```python
from build123d import *

# Parameters (mm, degrees)
F0_W     = 69.7
F0_H     = 17.7
F1_DEPTH = 1
F3_W     = 75.7
F3_H     = 23.7
F3_W_2   = 69.7
F3_H_2   = 17.7
F4_DEPTH = 1


with BuildPart() as f1:
    # F0 (on Top) → F1 (new body)
    with BuildSketch(Plane.XY):
        Rectangle(F0_W, F0_H)
    extrude(amount=F1_DEPTH)

    # F3 (on face) → F4 (join)
    with BuildSketch(Plane(origin=(0, 0, 0), x_dir=(1, 0, 0), z_dir=(0, 0, -1))):
        Rectangle(F3_W, F3_H)
        Rectangle(F3_W_2, F3_H_2, mode=Mode.SUBTRACT)
        Rectangle(F3_W_2, F3_H_2)
    extrude(amount=F4_DEPTH)


solid = f1.part
```
Verification items for the finished model (mm, model axes). Round coordinates to 2 decimals unless told otherwise and drop trailing zeros. Order: outer loops, then holes, each group sorted by start corner. A loop starts at its lowest first (then second) coordinate and runs counter-clockwise, first axis right, second up.
1) Cross-section at A-A, the plane x = 4.5. Record the cut outline in (y, z).
Geometry says:
outline: (-11.85, -1) - (11.85, -1) - (11.85, 0) - (8.85, 0) - (8.85, 1) - (-8.85, 1) - (-8.85, 0) - (-11.85, 0) - close
2) Cross-section at B-B, the plane y = 0.25. Record the cut outline in (x, z).
Geometry says:
outline: (-37.85, -1) - (37.85, -1) - (37.85, 0) - (34.85, 0) - (34.85, 1) - (-34.85, 1) - (-34.85, 0) - (-37.85, 0) - close
3) Depth check by flat-ended pin: pin 1 (1.1 mm diameter, centred on x = 15, z = 0.5, fed in from -Y); pin 2 (0.5 mm diameter, centred on y = 2.5, z = 0.5, fed in from +X). Enter the tip coordinate at first touch or a pass-through.
Geometry says:
pin 1: stops at y = -11.85
pin 2: stops at x = 34.85
4) Material ranges on line 1 (Y direction, x = 14, z = 0.1); line 2 (Z direction, x = 15.5, y = -10); line 3 (X direction, y = -2, z = 0.3), recorded low to high.
Geometry says:
line 1: y = -8.85 to 8.85
line 2: z = -1 to 0
line 3: x = -34.85 to 34.85
5) Cross-section at C-C, the plane z = 0.35. Record the cut outline in (x, y).
Geometry says:
outline: (-34.85, -8.85) - (34.85, -8.85) - (34.85, 8.85) - (-34.85, 8.85) - close
